Source: CAD feature listing. Evaluate the final solid. Frame: model axes, mm. Give positions to 0.01 mm unless a question says otherwise; leave off trailing zeros. Write each loop counter-clockwise with the first axis right and the second up, starting at its lowest first coordinate (ties: lowest second). Pieces come first, ordered by that corner, then holes. Notation, with made-up numbers: M -12,70.25 L -6,70.25 A34 ccw -6,100.25 Z; hole C 60,-22 d9. An arc over 180 degrees is marked long. Use CSV: the item, a comma, the result in double quotes. Start each with the question number.
Autodesk Fusion 360 part; units mm, degrees
sketch "Szkic1" plane through (0, 0, 0) normal (0, 0, 1) x (1, 0, 0)
  circle A0 centre (0, 0) radius 63.5
  line L0 (0, 4.2415) -> (0, 63.5)
  line L1 (4.2415, 0) -> (63.5, 0)
  line L2 (42.78, 42.78) -> (44.9013, 44.9013)
  line L3 (42.78, -42.78) -> (44.9013, -44.9013)
  line L4 (-42.78, -42.78) -> (-44.9013, -44.9013)
  circle A1 centre (44.9013, 44.9013) radius 3
  line L5 (46.9719, 42.7304) -> (4.2415, 0)
  line L6 (42.7304, 46.9719) -> (0, 4.2415)
  line L7 (-42.7304, 46.9719) -> (0, 4.2415)
  line L8 (-46.9719, 42.7304) -> (-4.2415, 0)
  circle A2 centre (-44.9013, 44.9013) radius 3
  line L9 (46.9719, -42.7304) -> (4.2415, 0)
  line L10 (42.7304, -46.9719) -> (0, -4.2415)
  circle A3 centre (44.9013, -44.9013) radius 3
  line L11 (-42.7304, -46.9719) -> (0, -4.2415)
  line L12 (-46.9719, -42.7304) -> (-4.2415, 0)
  circle A4 centre (-44.9013, -44.9013) radius 3
  circle A5 centre (-44.9013, 44.9013) radius 2
  circle A6 centre (44.9013, 44.9013) radius 2
  circle A7 centre (44.9013, -44.9013) radius 2
  circle A8 centre (-44.9013, -44.9013) radius 2
  dimension "d2" = 135
  dimension "d3" = 6
  dimension "d4" = 4
  dimension "d5" = 4
  dimension "d6" = 4
  dimension "d7" = 4
extrude "Wyciągnięcie proste1" add sketch "Szkic1" along normal blind 3 contours A0 L2 A1 A6 | A1 L5 L6 L7 L8 A2 L9 L10 A3 L11 L12 A4 | A0 A1 A6 | A0 A3 A7 | A0 L3 A3 A7 | A0 L2 A1 A6 | A0 L3 A3 A7 | A0 A4 A8 | A0 L4 A4 A8 | A0 A2 A5 | A0 A2 A5 | A0 L4 A4 A8
equation "d2 = 90 deg + 45 deg"
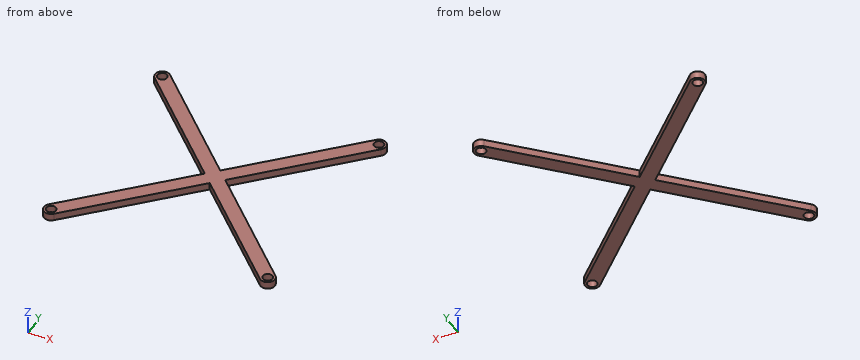
Item 1: Section C-C (y = -39.5). Return the cut outline in (x, z), plus the area to 3 significant figures.
Item 2: Section B-B (z = 1.95). Return the cut outline in (x, y).
Item 3: Material intervals for probe 1 along X at (y, z) = (-29.5, 1.2); probe 2 along X at (y, z) = (41, 2.2); probe 3 along Y at (x, z) = (39.5, 2.8), sorted ascending.
Item 4: Section D-D (y = 3). Return the cut outline in (x, z), plus the area to 3 significant figures.
Item 5: Contact query for flat-ended pins moving along their axis: pin 1 Ø10 at (x, y) = (17, 5) entering from +Z; pin 2 Ø1 at (y, z) = (-6, 1.5) entering from +X. Output: stop coordinate, or through.
Item 6: Section A-A (x = -20). Return the cut outline in (y, z), plus the area to 3 significant figures.
Output values:
1,outline,"M -43.74,0 L -35.26,0 L -35.26,3 L -43.74,3 Z; M 35.26,0 L 43.74,0 L 43.74,3 L 35.26,3 Z"
1,area,"50.9 mm2"
2,outline,"M -46.97,-42.73 A3 ccw long -42.73,-46.97 L 0,-4.24 L 42.73,-46.97 A3 ccw long 46.97,-42.73 L 4.24,0 L 46.97,42.73 A3 ccw long 42.73,46.97 L 0,4.24 L -42.73,46.97 A3 ccw long -46.97,42.73 L -4.24,0 Z; hole C -44.9,-44.9 d4; hole C -44.9,44.9 d4; hole C 44.9,-44.9 d4; hole C 44.9,44.9 d4"
3,probe 1,"x = -33.74 to -25.26, 25.26 to 33.74"
3,probe 2,"x = -45.24 to -36.76, 36.76 to 45.24"
3,probe 3,"y = -43.74 to -35.26, 35.26 to 43.74"
4,outline,"M -7.24,0 L 7.24,0 L 7.24,3 L -7.24,3 Z"
4,area,"43.4 mm2"
5,pin 1,"passes through"
5,pin 2,"stops at x = 10.74"
6,outline,"M -24.24,0 L -15.76,0 L -15.76,3 L -24.24,3 Z; M 15.76,0 L 24.24,0 L 24.24,3 L 15.76,3 Z"
6,area,"50.9 mm2"
